Build history of the part. All positions in model axes, mm. A direction names the side the tool comes from. Give positions to 0.01 mm unless a question says otherwise; leave off trailing zeros. Loops run counter-clockwise (first coordinate to the right, second up) from the corner with the lowest first, then second, coordinate; pieces in that order, holes last.
1) Flat gauge pins, fed straight in: P1, Ø1, axis at x = 64, y = -25.5, coming from the +Z side; P2, Ø24.5, axis at y = -27.5, z = 26.5, coming from the -X side; P3, Ø1, axis at x = 53, y = -31, coming from the +Z side; P4, Ø25, axis at x = 40, z = 60, coming from the +Y side. Where does each tip first touch, or does it go through?
2) Band-saw the part on B-B on x = 40. List the corners of the cut face in (y, z).
3) Two-plate mould, pull along Z, no slides. Class faces 1 (the flat face through (39, -32, 0)), 2 (the flat face through (0, -32, 5)), 3 (the flat face through (6.433, -4.93, 38.478)), 4 (the flat face through (35, -37, 21)): +Z half, -Z half, draft (parallel to the pull), parting line (faces both ways), or undercut.
4) Wall check: line 1 (Z direction, x = 40, y = -32); line 2 (Z direction, x = 33, y = -12.5); line 3 (Y direction, x = 29.5, z = 11). Give the ranges that are in metal, low to high.
5) Band-saw the part on C-C on z = 60. List the corners of the cut face in (x, y).
6) Band-saw the part on A-A on y = -44. List the corners of the cut face in (x, z).
7) 3-axis set-ups, long thin cutter, end or side, ignore diameter. For faces 5 (the flat face through (80, -32, 5)), 6 (the flat face through (18, -37, 10)), 7 (the flat face through (45, -37, 21)): which of +Z, -Z, +X, -X, +Y, -Y reach the whole face in a straight line?
8) Band-saw the part on D-D on z = 14.5. List the corners of the cut face in (x, y), then the cut area to 3 significant figures.
```python
from build123d import *

# Parameters (mm, degrees)
F0_R     = 14
F1_DEPTH = 64
F2_DEPTH = 10


with BuildPart() as f1:
    # F0 (on Front) → F1 (new body)
    with BuildSketch(Plane.XZ):
        with BuildLine():
            Line((0, 10), (0, 0))
            Line((0, 0), (80, 0))
            Line((80, 0), (80, 10))
            Line((80, 10), (45, 10))
            Line((45, 10), (45, 32.450045))
            ThreePointArc((45, 32.450045), (63.350892, 44.548921), (67.311856, 66.169485))
            ThreePointArc((67.311856, 66.169485), (40, 88), (12.688144, 66.169485))
            ThreePointArc((12.688144, 66.169485), (16.649108, 44.548921), (35, 32.450045))
            Line((35, 32.450045), (35, 10))
            Line((35, 10), (0, 10))
        make_face()
        with Locations((40, 60)):
            Circle(F0_R, mode=Mode.SUBTRACT)
    extrude(amount=F1_DEPTH)

    # F0 (on Front) → F2 (join)
    with BuildSketch(Plane.XZ):
        with BuildLine():
            Line((45, 10), (80, 10))
            Line((80, 10), (67.311856, 66.169485))
            ThreePointArc((67.311856, 66.169485), (63.350892, 44.548921), (45, 32.450045))
            Line((45, 32.450045), (45, 10))
        make_face()
        with BuildLine():
            Line((12.688144, 66.169485), (0, 10))
            Line((0, 10), (35, 10))
            Line((35, 10), (35, 32.450045))
            ThreePointArc((35, 32.450045), (16.649108, 44.548921), (12.688144, 66.169485))
        make_face()
    extrude(amount=F2_DEPTH)


solid = f1.part
```
Findings below:
1. P1: stops at z = 75.22
1. P2: stops at x = 21.77
1. P3: stops at z = 85.05
1. P4: passes through
2. outline: (-64, 0) - (0, 0) - (0, 46) - (-64, 46) - close; (-64, 74) - (0, 74) - (0, 88) - (-64, 88) - close
3. face 1: -Z half
3. face 2: draft
3. face 3: +Z half
3. face 4: undercut
4. line 1: z = 0 to 46, 74 to 88
4. line 2: z = 0 to 10, 32.89 to 47.88, 72.12 to 87.11
4. line 3: y = -10 to 0
5. outline: (11.29, -10) - (12, -10) - (12, -64) - (26, -64) - (26, 0) - (11.29, 0) - close; (54, -64) - (68, -64) - (68, -10) - (68.71, -10) - (68.71, 0) - (54, 0) - close
6. outline: (0, 0) - (80, 0) - (80, 10) - (45, 10) - (45, 32.45) arc R28 ccw to (67.31, 66.17) arc R28 ccw to (12.69, 66.17) arc R28 ccw to (35, 32.45) - (35, 10) - (0, 10) - close; hole circle Ø28 at (40, 60)
7. face 5: +Z, -Z, +X, +Y, -Y
7. face 6: -X, -Y
7. face 7: +X, -Y
8. outline: (1.02, -10) - (35, -10) - (35, -64) - (45, -64) - (45, -10) - (78.98, -10) - (78.98, 0) - (1.02, 0) - close
8. area: 1,320 mm2
